Here's how the part is built. I have some questions about the finished solid (model axes, mm). A direction names the side the tool comes from. Round coordinates to 2 decimals unless told otherwise and drop trailing zeros. Write each loop counter-clockwise with the first axis right and the second up, starting at its lowest first coordinate (ties: lowest second). Pieces come first, ordered by that corner, then holes. Notation, with made-up numbers: (40.5, -26.75) -> (79.5, -26.75) arc R28 cw to (79.5, -4.75) -> close; hole circle Ø11 at (60, 56). An arc over 180 degrees is marked (long way). Answer in a Markdown table with one row per item. Add a question column.
from build123d import *

# Parameters (mm, degrees)
SKETCH1_R           = 1.45
BOSS_EXTRUDE1_DEPTH = 3


with BuildPart() as part:
    # Sketch1 → Boss-Extrude1 (new body)
    with BuildSketch(Plane.XY.offset(1.9)):
        with BuildLine():
            Line((-13.026395415, 38.955911265), (-0.214852682, -8.857417136))
            ThreePointArc((-0.214852682, -8.857417136), (0.949961883, -10.375433033), (2.847009496, -10.625184089))
            Line((2.847009496, -10.625184089), (5.261824062, -9.978136476))
            Line((5.261824062, -9.978136476), (5.188879797, -9.705904774))
            Line((5.188879797, -9.705904774), (6.08761429, -9.187020173))
            ThreePointArc((6.08761429, -9.187020173), (5.919814799, -7.906537121), (5.481893659, -6.691622066))
            Line((5.481893659, -6.691622066), (5.414116812, -6.552658937))
            ThreePointArc((5.414116812, -6.552658937), (6.01040764, -6.01040764), (6.552658937, -5.414116812))
            Line((6.552658937, -5.414116812), (6.691622066, -5.481893659))
            ThreePointArc((6.691622066, -5.481893659), (7.906537121, -5.919814799), (9.187020173, -6.08761429))
            Line((9.187020173, -6.08761429), (9.86553871, -4.91238571))
            ThreePointArc((9.86553871, -4.91238571), (9.079978562, -3.887354604), (8.093270203, -3.054167872))
            Line((8.093270203, -3.054167872), (7.965092167, -2.967710696))
            ThreePointArc((7.965092167, -2.967710696), (8.210369523, -2.199961883), (8.381827508, -1.41243323))
            Line((8.381827508, -1.41243323), (8.536061531, -1.401648137))
            ThreePointArc((8.536061531, -1.401648137), (9.807169402, -1.173441441), (11, -0.678518537))
            Line((11, -0.678518537), (11, 0.678518537))
            ThreePointArc((11, 0.678518537), (9.807169402, 1.173441441), (8.536061531, 1.401648137))
            Line((8.536061531, 1.401648137), (8.381827508, 1.41243323))
            ThreePointArc((8.381827508, 1.41243323), (8.210369523, 2.199961883), (7.965092167, 2.967710696))
            Line((7.965092167, 2.967710696), (8.093270203, 3.054167872))
            ThreePointArc((8.093270203, 3.054167872), (9.079978562, 3.887354604), (9.86553871, 4.91238571))
            Line((9.86553871, 4.91238571), (9.187020173, 6.08761429))
            ThreePointArc((9.187020173, 6.08761429), (7.906537121, 5.919814799), (6.691622066, 5.481893659))
            Line((6.691622066, 5.481893659), (6.552658937, 5.414116812))
            ThreePointArc((6.552658937, 5.414116812), (6.01040764, 6.01040764), (5.414116812, 6.552658937))
            Line((5.414116812, 6.552658937), (5.481893659, 6.691622066))
            ThreePointArc((5.481893659, 6.691622066), (5.919814799, 7.906537121), (6.08761429, 9.187020173))
            Line((6.08761429, 9.187020173), (4.91238571, 9.86553871))
            ThreePointArc((4.91238571, 9.86553871), (3.887354604, 9.079978562), (3.054167872, 8.093270203))
            Line((3.054167872, 8.093270203), (2.967710696, 7.965092167))
            ThreePointArc((2.967710696, 7.965092167), (2.199961883, 8.210369523), (1.41243323, 8.381827508))
            Line((1.41243323, 8.381827508), (1.401648136, 8.536061531))
            ThreePointArc((1.401648136, 8.536061531), (1.173441441, 9.807169402), (0.678518537, 11))
            Line((0.678518537, 11), (-0.359250666, 11))
            Line((-0.359250666, 11), (-8.196766283, 40.250006491))
            ThreePointArc((-8.196766283, 40.250006491), (-11.258628462, 42.017773444), (-13.026395415, 38.955911265))
        make_face()
        with Locations((-10.611580849, 39.602958878)):
            Circle(SKETCH1_R, mode=Mode.SUBTRACT)
        Circle(SKETCH1_R, mode=Mode.SUBTRACT)
    extrude(amount=-BOSS_EXTRUDE1_DEPTH)


solid = part.part
Item 1: On a 3-axis mill with a long thin cutter (end or side, diameter ignored), from which of +Z, -Z, +X, -X, +Y, -Y can I reach the whole of each face in a straight line? I mean faces 4 (the cylindrical face through (6.02, 6, 0.42)), 5 (the cylindrical face through (7.889, -5.916, 0.421)), 6 (the cylindrical face through (9.067, 3.874, 0.421)), 7 (the flat face through (9.52, -5.51, 0.42)), 8 (the cylindrical face through (1.18, 9.79, 0.42)). Say none if no direction works.
Item 2: If we mould it in two halves opening along X, with no side actions, what happens to faces 1 (the flat face through (0, 11, 0)), 2 (the cylindrical face through (-1.45, 0.06, 0.42)), 3 (the cylindrical face through (5.924, -7.924, 0.421))? For each: pulls with the +X half, pulls with the -X half, needs draft (parallel to the pull), parting line crosses it, or undercut.
Item 3: If we section it at B-B on x = -7.5: Please give me the cut outline in (y, z), then the cut area to 3 significant figures.
Item 4: For P1, Ø10, axis at x = 4.5, y = 27.5, coming from the +Z side, with a flat end and sliding along its axis, tell me the tip position at first contact or that it passes through.
Item 5: If we section it at A-A on y = 0: Please give me the cut outline in (x, z).
Item 6: I need wall thicknesses on line 1 along Y through (x, z) = (6.5, 1.6); line 2 along Y through (x, z) = (0, 1.25); line 3 along X through (y, z) = (16, 1.4). Which ranges of each line are inside material? Lowest first, please. Write a range as from..to.
Item 7: If we section it at C-C on z = 1.25: Give the number of separate pieces and of enclosed holes in the cut face, then the cut area to 3 significant figures.
Item 8: If we section it at D-D on y = 17.5: Please give me the cut outline in (x, z), then the cut area to 3 significant figures.
Results list:
| question | item | result |
|---|---|---|
| 1 | face 4 | +Z, -Z |
| 1 | face 5 | +Z, -Z, -Y |
| 1 | face 6 | +Z, -Z, +X |
| 1 | face 7 | +Z, -Z, +X, -Y |
| 1 | face 8 | +Z, -Z, +Y |
| 2 | face 1 | needs draft |
| 2 | face 2 | undercut |
| 2 | face 3 | pulls with the +X half |
| 3 | outline | (18.33, -1.1) -> (37.65, -1.1) -> (37.65, 1.9) -> (18.33, 1.9) -> close |
| 3 | area | 58.0 mm² |
| 4 | P1 | through |
| 5 | outline | (-2.59, -1.1) -> (-1.45, -1.1) -> (-1.45, 1.9) -> (-2.59, 1.9) -> close; (1.45, -1.1) -> (11, -1.1) -> (11, 1.9) -> (1.45, 1.9) -> close |
| 6 | line 1 | -5.48..5.48 |
| 6 | line 2 | -9.4..-1.45, 1.45..11 |
| 6 | line 3 | -6.88..-1.7 |
| 7 | separate pieces | 1 |
| 7 | enclosed holes | 2 |
| 7 | area | 356 mm² |
| 8 | outline | (-7.28, -1.1) -> (-2.1, -1.1) -> (-2.1, 1.9) -> (-7.28, 1.9) -> close |
| 8 | area | 15.5 mm² |
